Check sheet for the modelled part. Datum: model origin and axes. Units: mm. Face numbers are marked on the shaded views. A direction names the side the tool comes from. Round coordinates to 2 decimals unless told otherwise and drop trailing zeros. Order: outer loops, then holes, each group sorted by start corner. A loop starts at its lowest first (then second) coordinate and runs counter-clockwise, first axis right, second up.
Q1. Mould release check, pull along Y, two halves, no side actions. Record for the marked faces 5, 6, 7 and 8: +Y half, -Y half, draft (parallel to the pull), parting line (faces both ways), or undercut.
Q2. Cross-section at B-B on y = -14. Record the cut outline in (x, z), then the cut area to 3 significant figures.
Q3. Cross-section at D-D on x = -18.5. Record the cut outline in (y, z).
Q4. Cross-section at C-C on x = -5.5. Record the cut outline in (y, z), then the cut area to 3 significant figures.
Q5. Cross-section at A-A on x = 9.5. Record the cut outline in (y, z).
Q6. Set-up check for the marked faces 1, 2, 3 and 4: record each of +Z, -Z, +X, -X, +Y, -Y from which the full face is reachable in a straight line by a thin tool's end or side.
Q7. Scan lines: probe 1 along X at (y, z) = (7.5, 6); probe 2 along Y at (x, z) = (-1.5, 1.5); probe 3 along X at (y, z) = (-7, 6.5). Record each from-to range of solid material in increasing order.
Q8. Depth check by flat-ended pin: P1, Ø1.6, axis at x = -27, z = 4, coming from the +Y side; P2, Ø3.5, axis at y = 24, z = 5, coming from the -X side; P3, Ø2, axis at y = -14, z = 4, coming from the +X side; P4, Ø12, axis at x = 6.5, y = -3, coming from the -Z side. Enter the tip coordinate at first touch or a pass-through.
from build123d import *

# Parameters (mm, degrees)
F0_W     = 11.3
F0_H     = 11.3
F0_H_2   = 18.7
F0_W_2   = 18.7
F0_H_3   = 15
F0_W_3   = 15
F1_DEPTH = 7
F2_R     = 3
F3_R     = 3


with BuildPart() as f1:
    # F0 (on Top) → F1 (new body)
    with BuildSketch(Plane.XY):
        with BuildLine():
            Line((-11.3, 9.8645831133), (-11.3, 0))
            ThreePointArc((-11.3, 0), (-7.9903066274, 7.9903066274), (0, 11.3))
            Line((0, 11.3), (0, 15))
            ThreePointArc((0, 15), (-6.2060959266, 13.6559281395), (-11.3, 9.8645831133))
        make_face()
        with BuildLine():
            Line((-15, 0), (-11.3, 0))
            Line((-11.3, 0), (-11.3, 9.8645831133))
            ThreePointArc((-11.3, 9.8645831133), (-14.0445719052, 5.2678268764), (-15, 0))
        make_face()
        with BuildLine():
            ThreePointArc((0, -11.3), (-7.9903066274, -7.9903066274), (-11.3, 0))
            Line((-11.3, 0), (-15, 0))
            ThreePointArc((-15, 0), (-13.6559281395, -6.2060959266), (-9.8645831133, -11.3))
            Line((-9.8645831133, -11.3), (0, -11.3))
        make_face()
        with BuildLine():
            ThreePointArc((-9.8645831133, -11.3), (-13.6559281395, -6.2060959266), (-15, 0))
            Line((-15, 0), (-21.7, 0))
            Line((-21.7, 0), (-21.7, -11.3))
            Line((-21.7, -11.3), (-9.8645831133, -11.3))
        make_face()
        with Locations((-27.35, -5.65)):
            Rectangle(F0_W, F0_H)
        with Locations((-27.35, 9.35)):
            Rectangle(F0_W, F0_H_2)
        with BuildLine():
            Line((-11.3, 21.7), (-11.3, 9.8645831133))
            ThreePointArc((-11.3, 9.8645831133), (-6.2060959266, 13.6559281395), (0, 15))
            Line((0, 15), (0, 21.7))
            Line((0, 21.7), (-11.3, 21.7))
        make_face()
        with Locations((-5.65, 27.35)):
            Rectangle(F0_W, F0_H)
        with Locations((9.35, 27.35)):
            Rectangle(F0_W_2, F0_H)
        with BuildLine():
            Line((21.7, 15), (0, 15))
            ThreePointArc((0, 15), (10.6066017178, 10.6066017178), (15, 0))
            Line((15, 0), (21.7, 0))
            Line((21.7, 0), (21.7, 15))
        make_face()
        with Locations((27.35, 7.5)):
            Rectangle(F0_W, F0_H_3)
        with Locations((27.35, -7.5)):
            Rectangle(F0_W, F0_H_3)
        with BuildLine():
            ThreePointArc((15, 0), (10.6066017178, -10.6066017178), (0, -15))
            Line((0, -15), (0, -21.7))
            Line((0, -21.7), (15, -21.7))
            Line((15, -21.7), (15, 0))
        make_face()
        with Locations((7.5, -27.35)):
            Rectangle(F0_W_3, F0_H)
        with Locations((-7.5, -27.35)):
            Rectangle(F0_W_3, F0_H)
        with BuildLine():
            ThreePointArc((11.3, 0), (7.9903066274, -7.9903066274), (0, -11.3))
            Line((0, -11.3), (0, -15))
            ThreePointArc((0, -15), (10.6066017178, -10.6066017178), (15, 0))
            Line((15, 0), (11.3, 0))
        make_face()
        with BuildLine():
            Line((0, -15), (0, -11.3))
            Line((0, -11.3), (-9.8645831133, -11.3))
            ThreePointArc((-9.8645831133, -11.3), (-5.2678268764, -14.0445719052), (0, -15))
        make_face()
        with BuildLine():
            Line((0, 15), (0, 11.3))
            ThreePointArc((0, 11.3), (7.9903066274, 7.9903066274), (11.3, 0))
            Line((11.3, 0), (15, 0))
            ThreePointArc((15, 0), (10.6066017178, 10.6066017178), (0, 15))
        make_face()
    extrude(amount=F1_DEPTH)

    # F2
    f2_edges = [f1.edges().sort_by_distance(p)[0] for p in [
        (21.7, 0, 3.5),
        (0, -21.7, 3.5),
        (-15, 0, 3.5),
        (0, 15, 3.5),
        (-11.3, 9.864583, 3.5),
        (0, -15, 3.5),
        (-9.864583, -11.3, 3.5),
        (15, 0, 3.5),
    ]]
    fillet(f2_edges, radius=F2_R)

    # F3
    f3_edges = [f1.edges().sort_by_distance(p)[0] for p in [
        (-33, -11.3, 3.5),
        (-15, -33, 3.5),
        (-33, 18.7, 3.5),
        (-21.7, 18.7, 3.5),
        (-15, -21.7, 3.5),
        (15, -33, 3.5),
        (21.7, -15, 3.5),
        (33, -15, 3.5),
        (33, 15, 3.5),
        (18.7, 21.7, 3.5),
        (18.7, 33, 3.5),
        (-11.3, 33, 3.5),
    ]]
    fillet(f3_edges, radius=F3_R)


solid = f1.part
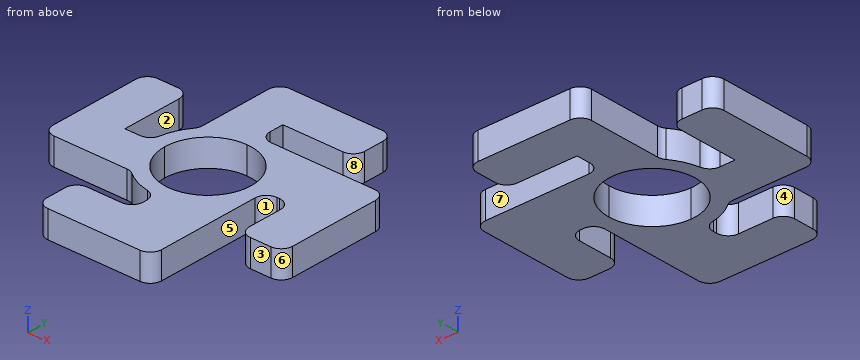
Results found:
1. face 5: draft
1. face 6: -Y half
1. face 7: undercut
1. face 8: undercut
2. outline: (-5.39, 0) - (15, 0) - (15, 7) - (-5.39, 7) - close; (22.46, 0) - (32.24, 0) - (32.24, 7) - (22.46, 7) - close
2. area: 211 mm2
3. outline: (-11.3, 0) - (0, 0) - (0, 7) - (-11.3, 7) - close
4. outline: (-33, 0) - (-21.7, 0) - (-21.7, 7) - (-33, 7) - close; (-13.96, 0) - (-9.87, 0) - (-9.87, 7) - (-13.96, 7) - close; (9.87, 0) - (33, 0) - (33, 7) - (9.87, 7) - close
4. area: 270 mm2
5. outline: (-33, 0) - (-6.12, 0) - (-6.12, 7) - (-33, 7) - close; (6.12, 0) - (15, 0) - (15, 7) - (6.12, 7) - close; (21.7, 0) - (33, 0) - (33, 7) - (21.7, 7) - close
6. face 1: +Z, -Z, -Y
6. face 2: +Z, -Z, +Y
6. face 3: +Z, -Z, +X, -Y
6. face 4: +Z, -Z, -X
7. probe 1: x = -33 to -21.7, -12.99 to -8.45, 8.45 to 33
7. probe 2: y = -33 to -21.3, -15.15 to -11.2, 11.2 to 33
7. probe 3: x = -33 to -8.87, 8.87 to 15, 21.7 to 33
8. P1: stops at y = 18.7
8. P2: stops at x = -11.3
8. P3: stops at x = 32.83
8. P4: stops at z = 0
